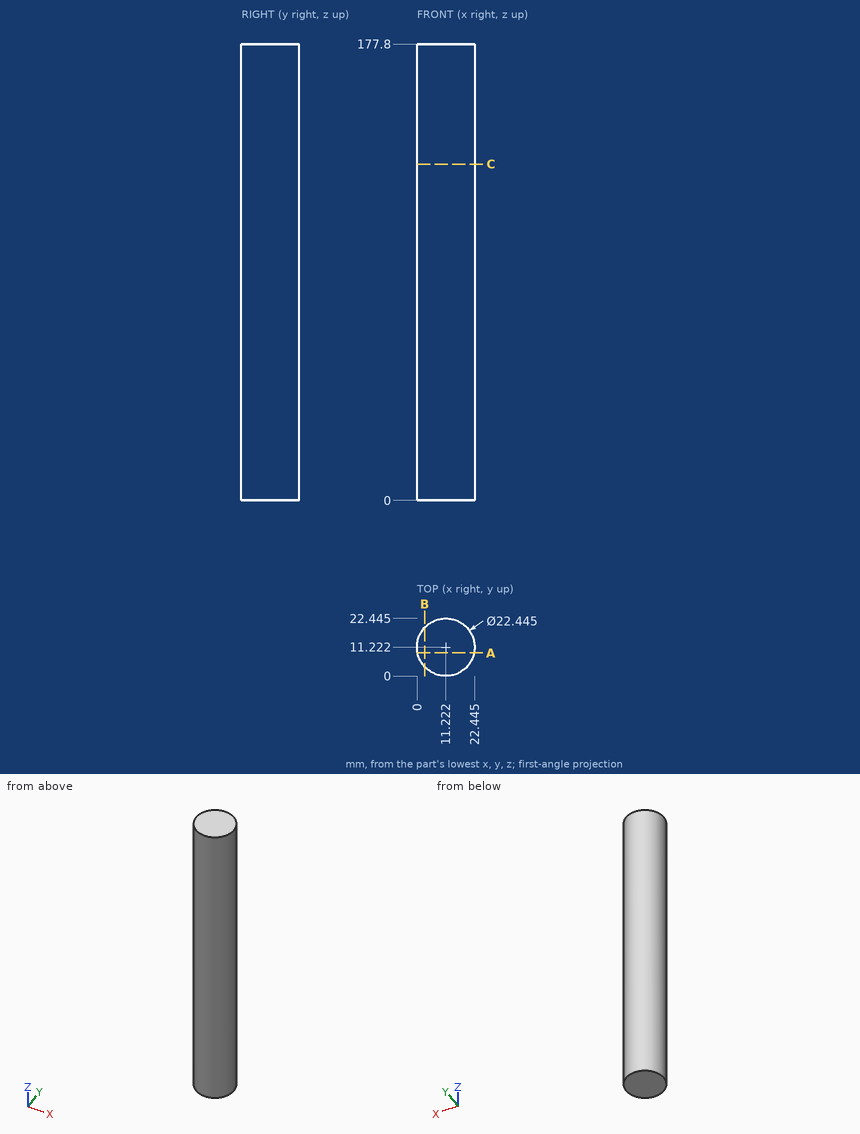
Study the drawing (mm; zero at the part's minimum x, y, z) and answer. Give positions to 0.01 mm unless a question says otherwise; leave off trailing zeros. Write each loop counter-clockwise with the first axis right and the second up, starting at its lowest first coordinate (ties: lowest second). Pieces come first, ordered by that corner, then holes.
(1) The part is cut by section A-A on y = 9. Write down the section's boundary in (x, z), plus the area to 3 significant figures.
Final values:
outline: (0.22, 0) - (22.22, 0) - (22.22, 177.8) - (0.22, 177.8) - close
area: 3,910 mm2
(2) The part is cut by section C-C on z = 131. Write down the section's boundary in (x, y) (1 decimal).
Final values:
outline: circle Ø22.4 at (11.2, 11.2)
(3) Straight lines are drawn through the part: line 1 (Y direction, x = 11.75, z = 98); line 2 (X direction, y = 19.25, z = 133) (1 decimal); line 3 (Y direction, x = 20, z = 53) (1 decimal). For each, find the intervals that lie inside material, in ascending order.
Final values:
line 1: y = 0.01 to 22.43
line 2: x = 3.4 to 19.1
line 3: y = 4.2 to 18.2
(4) The part is cut by section B-B on x = 3. Write down the section's boundary in (y, z) (1 decimal).
Final values:
outline: (3.6, 0) - (18.9, 0) - (18.9, 177.8) - (3.6, 177.8) - close
(5) Flat-ended cylindrical pins translate along their axes: pin 1 Ø8 at (y, z) = (13.5, 147) entering from +X (1 decimal); pin 2 Ø6 at (y, z) = (19, 143.5) entering from +X; pin 3 Ø12 at (x, z) = (3.5, 27.5) entering from +Y; pin 4 Ø1 at (y, z) = (7.5, 58.5) entering from +X. Find the tip coordinate at first contact, or state that the pin passes through.
Final values:
pin 1: stops at x = 22.4
pin 2: stops at x = 21.38
pin 3: stops at y = 22.31
pin 4: stops at x = 21.97
